from build123d import *

# Parameters (mm, degrees)
SZKIC1_W                    = 288
SZKIC1_H                    = 26
DODANIE_WYCI_GNI_CIE1_DEPTH = 6
SZKIC5_W                    = 40
SZKIC5_H                    = 6
WYTNIJ_WYCI_GNI_CIE3_DEPTH  = 6
SZYK_LINIOWY1_COUNT         = 4
SZYK_LINIOWY1_PITCH         = 91
WYTNIJ_WYCI_GNI_CIE4_DEPTH  = 6
SZYK_LINIOWY2_COUNT         = 2
SZYK_LINIOWY2_PITCH         = 91


with BuildPart() as part:
    # Szkic1 → Dodanie-wyciągnięcie1 (new body)
    with BuildSketch(Plane.XY):
        with Locations((-735.9, 7)):
            Rectangle(SZKIC1_W, SZKIC1_H)
    extrude(amount=-DODANIE_WYCI_GNI_CIE1_DEPTH)

    # Szkic5 → Wytnij-wyciągnięcie3 (cut)
    with BuildSketch(Plane.XY):
        with Locations((-872.9, -3)):
            Rectangle(SZKIC5_W, SZKIC5_H)
    wytnij_wyci_gni_cie3 = extrude(amount=-WYTNIJ_WYCI_GNI_CIE3_DEPTH, mode=Mode.SUBTRACT)

    # Szyk liniowy1: Wytnij-wyciągnięcie3 ×4
    with Locations(*[(i * SZYK_LINIOWY1_PITCH, 0, 0) for i in range(1, SZYK_LINIOWY1_COUNT)]):
        add(wytnij_wyci_gni_cie3, mode=Mode.SUBTRACT)

    # Szkic6 → Wytnij-wyciągnięcie4 (cut)
    with BuildSketch(Plane.XY):
        Polygon((-780.35, 0), (-783.45, 0), (-783.45, 4), (-784.825, 4), (-784.825, 6), (-783.45, 6), (-783.45, 6.5), (-780.35, 6.5), (-780.35, 6), (-778.975, 6), (-778.975, 4), (-780.35, 4), align=None)
    wytnij_wyci_gni_cie4 = extrude(amount=-WYTNIJ_WYCI_GNI_CIE4_DEPTH, mode=Mode.SUBTRACT)

    # Szyk liniowy2: Wytnij-wyciągnięcie4 ×2
    with Locations(*[(i * SZYK_LINIOWY2_PITCH, 0, 0) for i in range(1, SZYK_LINIOWY2_COUNT)]):
        add(wytnij_wyci_gni_cie4, mode=Mode.SUBTRACT)


solid = part.part
Build history of the part. All positions in model axes, mm. A direction names the side the tool comes from. Give positions to 0.01 mm unless a question says otherwise; leave off trailing zeros. Write each loop counter-clockwise with the first axis right and the second up, starting at its lowest first coordinate (ties: lowest second). Pieces come first, ordered by that corner, then holes. Notation, with made-up numbers: (29, 69) - (47, 69) arc R27 cw to (47, 108) - close; hole circle Ø2 at (80, 79.25). An arc over 180 degrees is marked (long way). Use one line per item in the form item = value. Start each with the question number.
1. 3-axis set-ups, long thin cutter, end or side, ignore diameter. For faces 5 (the face through (-738, 20, -3)), 6 (the face through (-879.9, 10, -3)), 7 (the face through (-606, 0, -3)), 8 (the face through (-702, 0, -3)), 9 (the face through (-867, 0, -3)): which of +Z, -Z, +X, -X, +Y, -Y reach the whole face in a straight line?
2. Probe line 1 (X direction, y = 3, z = -2.15); line 2 (X direction, y = -1, z = -4.6); line 3 (Y direction, x = -775.5, z = -3.6). List the from-to ranges inside material, lowest first. Write a range as [from, to].
3. Two-plate mould, pull along X, no slides. Class faces 1 (the face through (-801.9, -3, -3)), 2 (the face through (-852.9, -3, -3)), 3 (the face through (-793, 0, -3)), 4 (the face through (-738, 7, 0)): released by +X, released by -X, zero draft, split by the parting line, or undercut.
4. Drop flat-ended pins along their axis: pin 1 Ø1.8 at (y, z) = (-4, -2) entering from +X; pin 2 Ø0.7 at (x, z) = (-784, -3.5) entering from -Y. Give the stop position or say it passes through.
5. Band-saw the part on B-B on x = -706. Write the cut outline in (y, z), plus the area to 3 significant figures.
6. Band-saw the part on A-A on y = -3. Write the cut outline in (x, z), plus the area to 3 significant figures.
Conclusion:
q1.face_5 = +Z, -Z, +X, -X, +Y
q1.face_6 = +Z, -Z, -X, +Y, -Y
q1.face_7 = +Z, -Z, +X, -Y
q1.face_8 = +Z, -Z, -Y
q1.face_9 = +Z, -Z, -X, -Y
q2.line_1 = [-879.9, -783.45], [-780.35, -692.45], [-689.35, -591.9]
q2.line_2 = [-852.9, -801.9], [-761.9, -710.9], [-670.9, -619.9]
q2.line_3 = [0, 20]
q3.face_1 = undercut
q3.face_2 = released by -X
q3.face_3 = undercut
q3.face_4 = zero draft
q4.pin_1 = -619.9
q4.pin_2 = 0
q5.outline = (0, -6) - (20, -6) - (20, 0) - (0, 0) - close
q5.area = 120 mm²
q6.outline = (-852.9, -6) - (-801.9, -6) - (-801.9, 0) - (-852.9, 0) - close; (-761.9, -6) - (-710.9, -6) - (-710.9, 0) - (-761.9, 0) - close; (-670.9, -6) - (-619.9, -6) - (-619.9, 0) - (-670.9, 0) - close
q6.area = 918 mm²
